```python
from build123d import *

# Parameters (mm, degrees)
F0_W     = 37
F0_H     = 25
F2_DEPTH = 9.525
F1_R     = 5.25
F3_DEPTH = 12.5
F4_R     = 10
F6_D     = 11.1125
F6_DEPTH = 17.4625
F6_TIP   = 3.3385318145
F7_R     = 3.175


with BuildPart() as f2:
    # F0 (on Front) → F2 (new body, symmetric)
    with BuildSketch(Plane.XZ):
        Rectangle(F0_W, F0_H)
    extrude(amount=F2_DEPTH, both=True)

    # F1 (on Front) → F3 (cut, symmetric)
    with BuildSketch(Plane.XZ):
        with Locations((-9.525, 0)):
            Circle(F1_R)
    extrude(amount=F3_DEPTH, both=True, mode=Mode.SUBTRACT)

    # F4
    f4_edges = [f2.edges().sort_by_distance(p)[0] for p in [
        (-18.5, 0, -12.5),
    ]]
    fillet(f4_edges, radius=F4_R)

    # F6
    with Locations(Plane.YZ.offset(18.5)):
        with Locations((0, 0)):
            Hole(F6_D / 2, depth=F6_DEPTH)
            with Locations((0, 0, -(F6_DEPTH + F6_TIP / 2))):  # 118° drill point
                Cone(0, F6_D / 2, F6_TIP, mode=Mode.SUBTRACT)

    # F7
    f7_edges = [f2.edges().sort_by_distance(p)[0] for p in [
        (-18.5, 0, 12.5),
    ]]
    fillet(f7_edges, radius=F7_R)


solid = f2.part
```
Source: CAD feature listing. Evaluate the final solid. Frame: model axes, mm. Give positions to 0.01 mm unless a question says otherwise; leave off trailing zeros. Write each loop counter-clockwise with the first axis right and the second up, starting at its lowest first coordinate (ties: lowest second). Pieces come first, ordered by that corner, then holes.
1. Section query C-C (z = -8.5). Return the cut outline in (x, y) (3 decimals).
2. Pull-direction query (Z, two-part tool) for faces 1 (the face through (5, 0, -12.5)), 2 (the face through (9.65, -5.3, 1.67)), 3 (the face through (18.5, 0, -6)); classes: +Z half, -Z half, draft (parallel to the pull), parting line (faces both ways), or undercut.
3. Section query B-B (x = 10). Return the cut outline in (y, z) (1 decimal), then the cut area to 3 significant figures.
4. Material intervals for line 1 along Z through (x, y) = (14.25, 0); line 2 along Y through (x, z) = (11.5, 0) (3 decimals); line 3 along Y through (x, z) = (12.5, 2.75) (3 decimals), sorted ascending.
5. Section query A-A (y = 6.5). Return the cut outline in (x, z) (3 decimals), then the cut area to 3 significant figures.
Output values:
1. outline: (-16.5, -9.525) - (18.5, -9.525) - (18.5, 9.525) - (-16.5, 9.525) - close
2. face 1: -Z half
2. face 2: undercut
2. face 3: draft
3. outline: (-9.5, -12.5) - (9.5, -12.5) - (9.5, 12.5) - (-9.5, 12.5) - close; hole circle Ø11.1 at (0, 0)
3. area: 379 mm2
4. line 1: z = -12.5 to -5.56, 5.56 to 12.5
4. line 2: y = -9.525 to -5.556, 5.556 to 9.525
4. line 3: y = -9.525 to -4.828, 4.828 to 9.525
5. outline: (-18.5, -2.5) arc R10 ccw to (-8.5, -12.5) - (18.5, -12.5) - (18.5, 12.5) - (-15.325, 12.5) arc R3.175 ccw to (-18.5, 9.325) - close; hole circle Ø10.5 at (-9.525, 0)
5. area: 815 mm2
